The figure shows three views and two pictorial views of one solid part (mm, origin at its lowest corner). Answer the questions. Coordinates: 2 decimals unless noted, no trailing zeros. Order: outer loops, then holes, each group sorted by start corner. A loop starts at its lowest first (then second) coordinate and runs counter-clockwise, first axis right, second up. Notation, with made-up numbers: (39.5, 64) -> (82.5, 64) arc R16 ccw to (82.5, 95) -> close; hole circle Ø10 at (7, -7). An arc over 180 degrees is marked (long way). Write item = value, one per line.
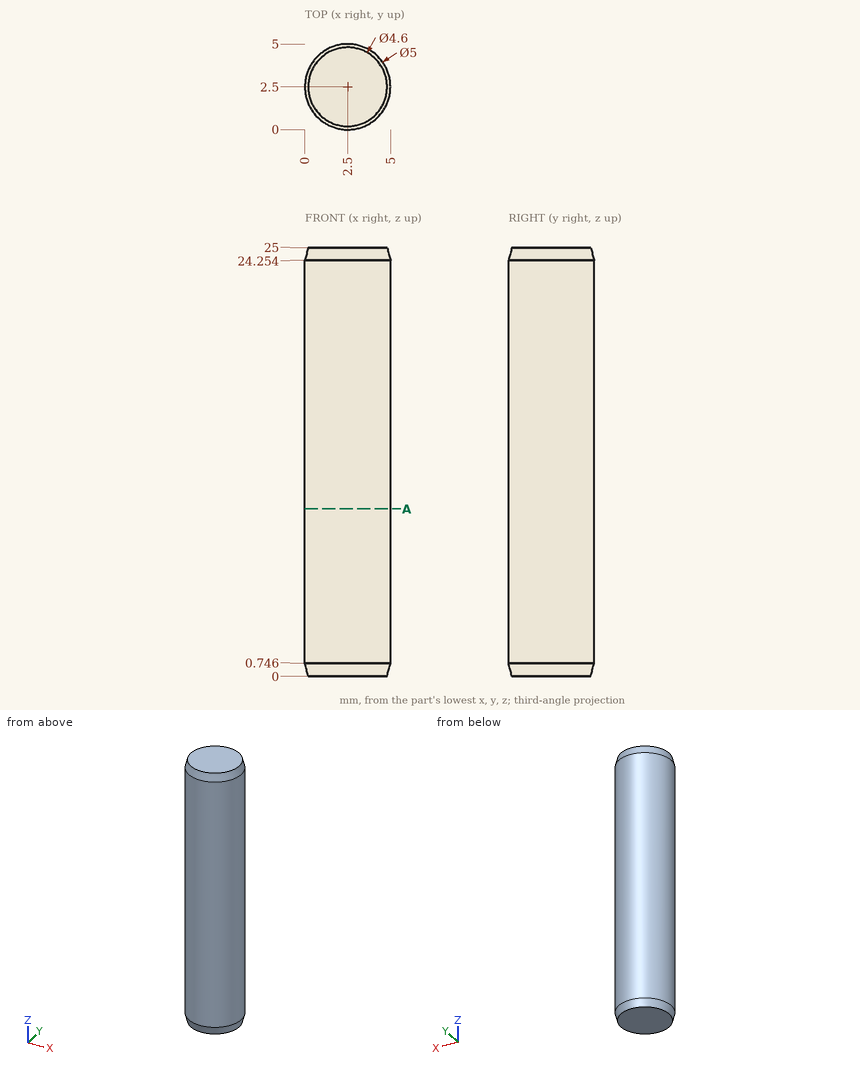
Q1. Find the intervals of material crossed by line 1 along Y through (x, z) = (2.6, 14.25); line 2 along X through (y, z) = (1.9, 11.25); line 3 along Y through (x, z) = (1.7, 11.25), in increasing order.
The answers:
line_1 = 0 to 5
line_2 = 0.07 to 4.93
line_3 = 0.13 to 4.87
Q2. Section A-A, the plane z = 9.75 is taken. Give the vertices of the cut face in (x, y).
The answers:
outline = circle Ø5 at (2.5, 2.5)
Q3. Each of these flat-tipped pins is pushed along its axis until it touches: pin 1 Ø1 at (x, z) = (1.5, 18) entering from +Y; pin 2 Ø1.5 at (x, z) = (3.5, 17.5) entering from +Y. Where does it stop, or does it pass through?
The answers:
pin_1 = 4.95
pin_2 = 4.99
